Geometry check sheet. Reference: the model listing, model coordinates, mm. Round coordinates to 2 decimals unless told otherwise and drop trailing zeros. Write each loop counter-clockwise with the first axis right and the second up, starting at its lowest first coordinate (ties: lowest second). Pieces come first, ordered by that corner, then holes. Notation, with made-up numbers: M 35.25,10 L 49.25,10 A11 ccw 49.25,17 Z; hole C 32.5,-1.5 d6. An arc over 180 degrees is marked long. Put each result on its own line as item: value. Start each with the question number.
(1) Section check A-A on x = 1.4. Record the cut outline in (y, z).
(2) Section check B-B on y = 15. Record the cut outline in (x, z), then the cut area to 3 significant figures.
(3) Gauge pin test, flat ends, axial feed: pin 1 (0.9 mm diameter, centred on x = 1.5, y = -2, fed in from +Z); pin 2 (4 mm diameter, centred on y = 0, z = -133.5, fed in from +X); pin 3 (0.9 mm diameter, centred on x = 2, y = -2, fed in from -Z); pin 4 (1 mm diameter, centred on x = 2, y = 6, fed in from +Z). Record the tip position at first contact, or that the pin passes through.
(4) Section check C-C on y = -12.5. Record the cut outline in (x, z), then the cut area to 3 significant figures.
(5) Material ranges on probe 1 along Y at (x, z) = (1.8, -133.5); probe 2 along Y at (x, z) = (1.3, 0); probe 3 along Z at (x, y) = (2.2, -6), recorded low to high.
Autodesk Inventor part; units mm, degrees
ref_plane "YZ Plane" through (0, 0, 0) normal (1, 0, 0) x (0, 1, 0)
ref_plane "XZ Plane" through (0, 0, 0) normal (0, 1, 0) x (-1, 0, 0)
ref_plane "XY Plane" through (0, 0, 0) normal (0, 0, 1) x (1, 0, 0)
sketch "Sketch1" plane through (0, 0, 0) normal (1, 0, 0) x (0, 1, 0)
  line L0 (0, 0) -> (0, -250) construction
  circle A0 centre (0, -250) radius 5
  arc A1 (0, -17.5) -> (17.5, 0) centre (0, 0) ccw construction
  arc A2 (0, -232.5) -> (-17.5, -250) centre (0, -250) ccw construction
  line L1 (17.5, 0) -> (17.5, -250)
  line L2 (-17.5, 0) -> (-17.5, -250)
  arc A3 (-17.5, 0) -> (0, -17.5) centre (0, 0) ccw construction
  arc A4 (17.5, 0) -> (-17.5, 0) centre (0, 0) ccw
  arc A5 (17.5, -250) -> (0, -232.5) centre (0, -250) ccw construction
  arc A6 (-17.5, -250) -> (17.5, -250) centre (0, -250) ccw
  line L3 (0, 0) -> (0, -80) construction
  line L4 (0, -80) -> (5, -80) construction
  line L5 (5, -80) -> (5, -83)
  line L6 (5, -83) -> (-5, -83) construction
  line L7 (-5, -83) -> (-5, -80)
  line L8 (-5, -80) -> (0, -80) construction
  line L9 (0, -250) -> (0, -150) construction
  line L10 (0, -150) -> (5, -150) construction
  line L11 (5, -150) -> (5, -147)
  line L12 (5, -147) -> (-5, -147) construction
  line L13 (-5, -147) -> (-5, -150)
  line L14 (0, -150) -> (-5, -150) construction
  line L15 (0, -250) -> (0, -125) construction
  circle A7 centre (0, -125) radius 3.5
  line L16 (0, -125) -> (0, -133.5) construction
  line L17 (0, -125) -> (0, -116.5) construction
  circle A8 centre (0, -116.5) radius 1.5
  circle A9 centre (0, -133.5) radius 1.5
  line L18 (7.5, 0) -> (13.5, 0) construction
  arc A10 (2.5, -6.8053) -> (-2.5, -6.8053) centre (0, 0) ccw
  line L19 (0, -7.25) -> (2.5, -7.25) construction
  line L20 (2.5, -7.25) -> (-2.5, -7.25) construction
  line L21 (-2.5, -7.25) -> (-2.5, -8.75)
  line L22 (-2.5, -8.75) -> (2.5, -8.75)
  line L23 (2.5, -8.75) -> (2.5, -7.25)
  line L24 (2.5, -7.25) -> (2.5, -6.8053)
  line L25 (-2.5, -7.25) -> (-2.5, -6.8053)
  arc A11 (0, -7.25) -> (2.5, -6.8053) centre (0, 0) ccw construction
  arc A12 (-2.5, -6.8053) -> (0, -7.25) centre (0, 0) ccw construction
  line L26 (-5, -80) -> (-5, -79.75)
  line L27 (-5, -79.75) -> (5, -79.75)
  line L28 (5, -79.75) -> (5, -80)
  line L29 (5, -83) -> (5, -83.25)
  line L30 (5, -83.25) -> (-5, -83.25)
  line L31 (-5, -83.25) -> (-5, -83)
  line L32 (5, -150) -> (5, -150.25)
  line L33 (5, -150.25) -> (-5, -150.25)
  line L34 (-5, -150.25) -> (-5, -150)
  line L35 (-5, -147) -> (-5, -146.75)
  line L36 (-5, -146.75) -> (5, -146.75)
  line L37 (5, -146.75) -> (5, -147)
  dimension "d1" = 250
  dimension "d2" = 10
  dimension "d3" = 35
  dimension "d4" = 35
  dimension "d5" = 80
  dimension "d6" = 5
  dimension "d7" = 3
  dimension "d8" = 10
  dimension "d9" = 100
  dimension "d10" = 3
  dimension "d11" = 10
  dimension "d21" = 125
  dimension "d22" = 7
  dimension "d23" = 8.5
  dimension "d24" = 8.5
  dimension "d25" = 3
  dimension "d26" = 3
  dimension "d29" = 14.5
  dimension "d30" = 2.5
  dimension "d31" = 5
  dimension "d32" = 1.5
  dimension "d33" = 0.25
  dimension "d34" = 10
  dimension "d35" = 0.25
  dimension "d36" = 0.25
  dimension "d37" = 10
  dimension "d38" = 0.25
  dimension "d39" = 0.25
  dimension "d40" = 10
  dimension "d41" = 0.25
  dimension "d42" = 0.25
  dimension "d43" = 10
  dimension "d44" = 0.25
extrude "Extrusion1" add sketch "Sketch1" along normal blind 3
properties part number "brazo2" material "PMMA Plastic"
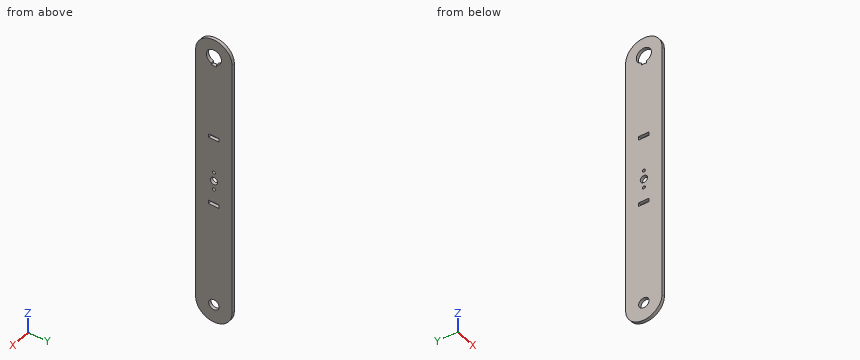
Answers follow:
1. outline: M -17.5,-250 A17.5 ccw 17.5,-250 L 17.5,0 A17.5 ccw -17.5,0 Z; hole C 0,-250 d10; hole M -5,-150.25 L 5,-150.25 L 5,-146.75 L -5,-146.75 Z; hole M -5,-83.25 L 5,-83.25 L 5,-79.75 L -5,-79.75 Z; hole C 0,-125 d7; hole M -2.5,-8.75 L 2.5,-8.75 L 2.5,-6.81 A7.25 ccw long -2.5,-6.81 Z; hole C 0,-133.5 d3; hole C 0,-116.5 d3
2. outline: M 0,-259.01 L 3,-259.01 L 3,9.01 L 0,9.01 Z
2. area: 804 mm^2
3. pin 1: stops at z = 17.43
3. pin 2: stops at x = 3
3. pin 3: stops at z = -267.43
3. pin 4: stops at z = 16.61
4. outline: M 0,-262.25 L 3,-262.25 L 3,12.25 L 0,12.25 Z
4. area: 823 mm^2
5. probe 1: y = -17.5 to -1.5, 1.5 to 17.5
5. probe 2: y = -17.5 to -7.25, 7.25 to 17.5
5. probe 3: z = -266.44 to -4.07, 4.07 to 16.44
